Part model, mm, in its own coordinate system. A direction names the side the tool comes from. Round coordinates to 2 decimals unless told otherwise and drop trailing zeros. Loops run counter-clockwise (first coordinate to the right, second up) from the corner with the lowest first, then second, coordinate; pieces in that order, holes last. Notation, with made-up numbers: (53, -21) - (92, -21) arc R22 cw to (92, -5) - close; hole circle Ø6 at (27, 70.25). An arc over 180 degrees is marked (long way). Write each question's results on one line, items separated by ' | '. Start each with the question number.
(1) Cut at A-A, the plane x = -30.48. List the corners of the cut face in (y, z) (3 decimals).
(2) Cut at B-B, the plane y = 6. List the corners of the cut face in (x, z) (1 decimal).
(3) Cut at D-D, the plane y = 0. Give the number of separate pieces and of enclosed holes in the cut face, then the cut area to 3 significant figures.
(4) Mould opens along X. For faces 5 (the face through (34, 0, 11.303)), 6 (the face through (-30, -2, 3.048)), 7 (the face through (-26.352, 0, 14)) say: released by +X, released by -X, zero draft, split by the parting line, or undercut.
(5) Flat gauge pins, fed straight in: P1, Ø4.5, axis at x = -30.48, y = 0, coming from the -Z side; P2, Ø8, axis at x = -31.5, y = 4, coming from the +Z side; P3, Ø1.6, axis at y = 2.5, z = 14.5, coming from the +X side; P4, Ø5.5, axis at x = 0, z = 8.255, coming from the +Y side. Where does each tip first touch, or does it go through?
(6) Drill centre lines: L1, parallel to X at y = 0, z = 4.25; L2, parallel to X at y = 0, z = 0.9; L3, parallel to X at y = 0, z = 6.75. Where is each one in solid material? Low to high.
(7) Tool access for faces 1 (the face through (41.202, 1.283, 1.545)), 2 (the face through (1, 8.255, 4)), 3 (the face through (26.352, 0, 14)), 4 (the face through (-0.1, -1.905, 4.6)): list every direction of +Z, -Z, +X, -X, +Y, -Y with a clear straight run to the whole face (end or side of a thin tool).
(8) Cut at C-C, the plane z = 9. List the corners of the cut face in (x, y) (1 decimal).
Autodesk Inventor part; units mm, degrees
ref_plane "Work Plane1" through (0, -8.255, 0) normal (1, 0, 0) x (0, 0, -1)
ref_plane "YZ Plane" through (0, 0, 0) normal (1, 0, 0) x (0, 1, 0)
ref_plane "XZ Plane" through (0, 0, 0) normal (0, 1, 0) x (-1, 0, 0)
sketch "Sketch2" plane through (0, 0, 0) normal (0, 0, 1) x (1, 0, 0)
  line L0 (-42.8625, -8.255) -> (42.8625, -8.255)
  line L1 (42.8625, -8.255) -> (42.8625, 8.255)
  line L2 (42.8625, 8.255) -> (-42.8625, 8.255)
  line L3 (-42.8625, 8.255) -> (-42.8625, -8.255)
  line L4 (-42.8625, -8.255) -> (42.8625, 8.255) construction
  line L5 (42.8625, -8.255) -> (-42.8625, 8.255) construction
  point P0 (0, 0)
  dimension "bar_length" = 85.725
  dimension "bar_width" = 16.51
extrude "Extrusion1" add sketch "Sketch2" along normal blind 16.51
ref_plane "Work Plane1" through (0, -8.255, 0) normal (1, 0, 0) x (0, 0, -1)
sketch "Sketch5" plane through (0, 0, 0) normal (0, 0, -1) x (-1, 0, 0)
  line L0 (42.8625, -8.255) -> (-42.8625, -8.255) construction
  line L1 (42.8625, 8.255) -> (42.8625, -8.255) construction
  line L2 (-42.8625, 8.255) -> (42.8625, 8.255) construction
  line L3 (-42.8625, -8.255) -> (-42.8625, 8.255) construction
  line L4 (-42.8625, -8.255) -> (-26.3525, -8.255) construction
  line L5 (-26.3525, -8.255) -> (-26.3525, 8.255) construction
  line L6 (-26.3525, 8.255) -> (-42.8625, 8.255) construction
  line L7 (-42.8625, 8.255) -> (-42.8625, -8.255) construction
  line L8 (-34.6075, -8.255) -> (-34.6075, 8.255) construction
  line L9 (-38.735, -8.255) -> (-38.735, 8.255) construction
  line L10 (-30.48, -8.255) -> (-30.48, 8.255) construction
  line L11 (-34.6075, -8.255) -> (-34.6075, 8.255) construction
  point P0 (0, 0)
  point P1 (-30.48, 0)
  point P2 (-38.735, 0)
  dimension "d10" = 16.51
  dimension "d11" = 16.51
  dimension "d14" = 4.1275
  dimension "d17" = 4.1275
hole "Hole1" at (30.48, 0, 0) at (38.735, 0, 0) direction (0, 0, 1) diameter 3.4544 end through all counterbore diameter 5.5626 counterbore depth 3.048
sketch "Sketch4" plane through (0, 0, 16.51) normal (0, 0, 1) x (1, 0, 0)
  line L0 (-42.8625, -8.255) -> (42.8625, -8.255) construction
  line L1 (42.8625, -8.255) -> (42.8625, 8.255) construction
  line L2 (42.8625, 8.255) -> (-42.8625, 8.255) construction
  line L3 (-42.8625, 8.255) -> (-42.8625, -8.255) construction
  line L4 (42.8625, -8.255) -> (26.3525, -8.255)
  line L5 (26.3525, -8.255) -> (26.3525, 8.255)
  line L6 (26.3525, 8.255) -> (42.8625, 8.255)
  line L7 (42.8625, 8.255) -> (42.8625, -8.255)
  circle A0 centre (38.735, 0) radius 1.7272
  point P0 (0, 0)
  dimension "d6" = 16.51
  dimension "d7" = 16.51
extrude "Extrusion2" cut sketch "Sketch4" against normal blind 5.207 contours L4 L5 L6 L7 | A0
mirror "Mirror2" about plane through (0, -8.255, 0) normal (1, 0, 0) of "Hole1", "Extrusion2"
sketch "Sketch7" plane through (-42.8625, -8.255, 0) normal (0, -1, 0) x (1, 0, 0)
  line L0 (0, 0) -> (85.725, 0)
  line L1 (85.725, 0) -> (85.725, 11.303)
  line L2 (16.51, 16.51) -> (69.215, 16.51)
  line L3 (0, 0) -> (0, 11.303)
  line L4 (55.5625, 8.255) -> (42.8625, 8.255)
  line L5 (0, 16.51) -> (85.725, 16.51)
  line L6 (42.8625, 8.255) -> (30.1625, 8.255)
  line L7 (85.725, 8.255) -> (0, 8.255) construction
  line L8 (42.8625, 0) -> (42.8625, 16.51) construction
  line L9 (16.51, 16.51) -> (16.51, 11.303)
  line L10 (16.51, 11.303) -> (0, 11.303)
  line L11 (85.725, 11.303) -> (69.215, 11.303)
  line L12 (69.215, 11.303) -> (69.215, 16.51)
  dimension "d48" = 12.7
hole "Hole6" at (0, -8.255, 8.255) direction (0, 1, 0) diameter 6.7564 end through all counterbore diameter 11.1252 counterbore depth 6.35
equation "\"d2\" = bar_width"
equation "\"d14\" = 0.5 * hole_spacing"
equation "\"d17\" = 0.5 * hole_spacing"
equation "\"hole_spacing\" = 8.255"
properties part number "hph_C_001"
A:
1) outline: (-8.255, 0) - (-2.781, 0) - (-2.781, 3.048) - (-1.727, 3.048) - (-1.727, 11.303) - (-8.255, 11.303) - close; (1.727, 3.048) - (2.781, 3.048) - (2.781, 0) - (8.255, 0) - (8.255, 11.303) - (1.727, 11.303) - close
2) outline: (-42.9, 0) - (42.9, 0) - (42.9, 11.3) - (26.4, 11.3) - (26.4, 16.5) - (-26.4, 16.5) - (-26.4, 11.3) - (-42.9, 11.3) - close; hole circle Ø6.8 at (0, 8.3)
3) separate pieces: 5 | enclosed holes: 1 | area: 1,030 mm2
4) face 5: zero draft | face 6: undercut | face 7: released by -X
5) P1: z = 3.05 | P2: z = 11.3 | P3: x = 26.35 | P4: through
6) L1: -42.86 to -40.46, -37.01 to -32.21, -28.75 to 28.75, 32.21 to 37.01, 40.46 to 42.86 | L2: -42.86 to -41.52, -35.95 to -33.26, -27.7 to 27.7, 33.26 to 35.95, 41.52 to 42.86 | L3: -42.86 to -40.46, -37.01 to -32.21, -28.75 to -3.02, 3.02 to 28.75, 32.21 to 37.01, 40.46 to 42.86
7) face 1: -Z | face 2: +Z, -Z, +X, -X, +Y | face 3: +Z, +X, +Y, -Y | face 4: -Y
8) outline: (-42.9, -8.3) - (-5.5, -8.3) - (-5.5, -1.9) - (-3.3, -1.9) - (-3.3, 8.3) - (-42.9, 8.3) - close; (3.3, -1.9) - (5.5, -1.9) - (5.5, -8.3) - (42.9, -8.3) - (42.9, 8.3) - (3.3, 8.3) - close; hole circle Ø3.5 at (-38.7, 0); hole circle Ø3.5 at (-30.5, 0); hole circle Ø3.5 at (30.5, 0); hole circle Ø3.5 at (38.7, 0)
